```python
from build123d import *

# Parameters (mm, degrees)
BOSS_EXTRUDE1_DEPTH      = 30
BOSS_EXTRUDE1_DEPTH_BACK = 70
CUT_EXTRUDE1_REACH       = 92
SKETCH2_R                = 4.5
SKETCH2_R_2              = 5.1
SKETCH2_R_3              = 3.8
SKETCH5_W                = 20
SKETCH5_H                = 20
CUT_EXTRUDE2_DEPTH       = 91
CUT_EXTRUDE3_REACH       = 92
SKETCH7_W                = 20
SKETCH7_H                = 20
SKETCH8_R                = 5
SKETCH8_R_2              = 4.1
SKETCH8_R_3              = 3.8
CUT_EXTRUDE6_DEPTH       = 10
SKETCH9_W                = 20
SKETCH9_H                = 20
SKETCH9_W_2              = 3
SKETCH9_H_2              = 3
CUT_EXTRUDE7_DEPTH       = 81
BOSS_EXTRUDE2_DEPTH      = 80


with BuildPart() as part:
    # Sketch1 → Boss-Extrude1 (new body, two sides)
    with BuildSketch(Plane(origin=(0, 0, 0), x_dir=(1, 0, 0), z_dir=(0, 1, 0))) as boss_extrude1_sk:
        with BuildLine():
            Line((-25, 45), (25, 45))
            ThreePointArc((25, 45), (39.142135624, 39.142135624), (45, 25))
            Line((45, 25), (45, -25))
            ThreePointArc((45, -25), (39.142135624, -39.142135624), (25, -45))
            Line((25, -45), (-25, -45))
            ThreePointArc((-25, -45), (-39.142135624, -39.142135624), (-45, -25))
            Line((-45, -25), (-45, 25))
            ThreePointArc((-45, 25), (-39.142135624, 39.142135624), (-25, 45))
        make_face()
        with BuildLine():
            Line((-25, 35), (25, 35))
            ThreePointArc((25, 35), (32.071067812, 32.071067812), (35, 25))
            Line((35, 25), (35, -25))
            ThreePointArc((35, -25), (32.071067812, -32.071067812), (25, -35))
            Line((25, -35), (-25, -35))
            ThreePointArc((-25, -35), (-32.071067812, -32.071067812), (-35, -25))
            Line((-35, -25), (-35, 25))
            ThreePointArc((-35, 25), (-32.071067812, 32.071067812), (-25, 35))
        make_face(mode=Mode.SUBTRACT)
    extrude(amount=BOSS_EXTRUDE1_DEPTH)
    extrude(boss_extrude1_sk.sketch, amount=-BOSS_EXTRUDE1_DEPTH_BACK)

    # Sketch2 → Cut-Extrude1 (cut, up to next)
    with BuildSketch(Plane(origin=(45, 0, 0), x_dir=(0, 0, -1), z_dir=(1, 0, 0)), mode=Mode.PRIVATE) as cut_extrude1_sk1:
        with Locations((-0.001556395, 0)):
            Circle(SKETCH2_R)
    cut_extrude1_tool1 = extrude(cut_extrude1_sk1.sketch, amount=-CUT_EXTRUDE1_REACH, mode=Mode.PRIVATE) & part.part
    add(cut_extrude1_tool1.solids().sort_by_distance((45, 0, 0.001556))[0], mode=Mode.SUBTRACT)
    # Sketch2 → Cut-Extrude1 (cut, up to next)
    with BuildSketch(Plane(origin=(45, 0, 0), x_dir=(0, 0, -1), z_dir=(1, 0, 0)), mode=Mode.PRIVATE) as cut_extrude1_sk2:
        with Locations((-0.001556395, -35)):
            Circle(SKETCH2_R_2)
    cut_extrude1_tool2 = extrude(cut_extrude1_sk2.sketch, amount=-CUT_EXTRUDE1_REACH, mode=Mode.PRIVATE) & part.part
    add(cut_extrude1_tool2.solids().sort_by_distance((45, -35, 0.001556))[0], mode=Mode.SUBTRACT)
    # Sketch2 → Cut-Extrude1 (cut, up to next)
    with BuildSketch(Plane(origin=(45, 0, 0), x_dir=(0, 0, -1), z_dir=(1, 0, 0)), mode=Mode.PRIVATE) as cut_extrude1_sk3:
        with Locations((15.998443605, -35)):
            Circle(SKETCH2_R_3)
    cut_extrude1_tool3 = extrude(cut_extrude1_sk3.sketch, amount=-CUT_EXTRUDE1_REACH, mode=Mode.PRIVATE) & part.part
    add(cut_extrude1_tool3.solids().sort_by_distance((45, -35, -15.998444))[0], mode=Mode.SUBTRACT)
    # Sketch2 → Cut-Extrude1 (cut, up to next)
    with BuildSketch(Plane(origin=(45, 0, 0), x_dir=(0, 0, -1), z_dir=(1, 0, 0)), mode=Mode.PRIVATE) as cut_extrude1_sk4:
        with Locations((-16.001556395, -35)):
            Circle(SKETCH2_R_3)
    cut_extrude1_tool4 = extrude(cut_extrude1_sk4.sketch, amount=-CUT_EXTRUDE1_REACH, mode=Mode.PRIVATE) & part.part
    add(cut_extrude1_tool4.solids().sort_by_distance((45, -35, 16.001556))[0], mode=Mode.SUBTRACT)
    # Sketch2 → Cut-Extrude1 (cut, up to next)
    with BuildSketch(Plane(origin=(45, 0, 0), x_dir=(0, 0, -1), z_dir=(1, 0, 0)), mode=Mode.PRIVATE) as cut_extrude1_sk5:
        with BuildLine():
            ThreePointArc((20.848443603, 0), (18.248443605, 2.599999998), (15.648443602, 0))
            ThreePointArc((15.648443602, 0), (18.248443605, -2.600000003), (20.848443603, 0))
        make_face()
    cut_extrude1_tool5 = extrude(cut_extrude1_sk5.sketch, amount=-CUT_EXTRUDE1_REACH, mode=Mode.PRIVATE) & part.part
    add(cut_extrude1_tool5.solids().sort_by_distance((45, 0, -18.248444))[0], mode=Mode.SUBTRACT)
    # Sketch2 → Cut-Extrude1 (cut, up to next)
    with BuildSketch(Plane(origin=(45, 0, 0), x_dir=(0, 0, -1), z_dir=(1, 0, 0)), mode=Mode.PRIVATE) as cut_extrude1_sk6:
        with BuildLine():
            ThreePointArc((-15.651556392, 0), (-18.251556395, 2.600000003), (-20.851556393, 0))
            ThreePointArc((-20.851556393, 0), (-18.251556395, -2.599999997), (-15.651556392, 0))
        make_face()
    cut_extrude1_tool6 = extrude(cut_extrude1_sk6.sketch, amount=-CUT_EXTRUDE1_REACH, mode=Mode.PRIVATE) & part.part
    add(cut_extrude1_tool6.solids().sort_by_distance((45, 0, 18.251556))[0], mode=Mode.SUBTRACT)

    # Sketch5 → Cut-Extrude2 (cut, through all)
    with BuildSketch(Plane(origin=(45, 0, 0), x_dir=(0, 0, -1), z_dir=(1, 0, 0))):
        with Locations((35, 20)):
            Rectangle(SKETCH5_W, SKETCH5_H)
    extrude(amount=-CUT_EXTRUDE2_DEPTH, mode=Mode.SUBTRACT)

    # Sketch7 → Cut-Extrude3 (cut, up to next)
    with BuildSketch(Plane.XY.offset(45), mode=Mode.PRIVATE) as cut_extrude3_sk1:
        with Locations((-35, 20)):
            Rectangle(SKETCH7_W, SKETCH7_H)
    cut_extrude3_tool1 = extrude(cut_extrude3_sk1.sketch, amount=-CUT_EXTRUDE3_REACH, mode=Mode.PRIVATE) & part.part
    add(cut_extrude3_tool1.solids().sort_by_distance((-35, 20, 45))[0], mode=Mode.SUBTRACT)

    # Sketch8 → Cut-Extrude6 (cut)
    with BuildSketch(Plane.XY.offset(45)):
        with Locations((640, -50.6)):
            Circle(SKETCH8_R)
        with Locations((640, -15.6)):
            Circle(SKETCH8_R)
        with Locations((0, -15.6)):
            Circle(SKETCH8_R_2)
        with Locations((0, -50.6)):
            Circle(SKETCH8_R)
        with Locations((-16, -50.6)):
            Circle(SKETCH8_R_3)
        with Locations((16, -50.6)):
            Circle(SKETCH8_R_3)
        with BuildLine():
            ThreePointArc((-15.649999997, -15.6), (-18.25, -12.999999997), (-20.849999998, -15.6))
            ThreePointArc((-20.849999998, -15.6), (-18.25, -18.199999997), (-15.649999997, -15.6))
        make_face()
        with BuildLine():
            ThreePointArc((20.849999998, -15.6), (18.25, -13.000000002), (15.649999997, -15.6))
            ThreePointArc((15.649999997, -15.6), (18.25, -18.200000003), (20.849999998, -15.6))
        make_face()
    extrude(amount=-CUT_EXTRUDE6_DEPTH, mode=Mode.SUBTRACT)

    # Sketch9 → Cut-Extrude7 (cut, through all)
    with BuildSketch(Plane(origin=(0, 10, 0), x_dir=(1, 0, 0), z_dir=(0, 1, 0))):
        with Locations((-35, 35)):
            Rectangle(SKETCH9_W, SKETCH9_H)
        with Locations((-36.5, 15)):
            Rectangle(SKETCH9_W_2, SKETCH9_H)
        with Locations((-15, 36.5)):
            Rectangle(SKETCH9_W, SKETCH9_H_2)
    extrude(amount=-CUT_EXTRUDE7_DEPTH, mode=Mode.SUBTRACT)

    # Sketch10 → Boss-Extrude2 (add)
    with BuildSketch(Plane(origin=(0, 10, 0), x_dir=(1, 0, 0), z_dir=(0, 1, 0))):
        with BuildLine():
            Line((-25, 45), (-25, 25))
            Line((-25, 25), (-45, 25))
            Line((-45, 25), (-45, 15))
            Line((-45, 15), (-25, 15))
            ThreePointArc((-25, 15), (-17.928932188, 17.928932188), (-15, 25))
            Line((-15, 25), (-15, 45))
            Line((-15, 45), (-25, 45))
        make_face()
    extrude(amount=-BOSS_EXTRUDE2_DEPTH)


solid = part.part
```
Verification items for the finished model (mm, model axes). A direction names the side the tool comes from. Coordinates: 2 decimals unless noted, no trailing zeros. Write each loop counter-clockwise with the first axis right and the second up, starting at its lowest first coordinate (ties: lowest second). Pieces come first, ordered by that corner, then holes. Notation, with made-up numbers: M 44,-7 L 90,-7 A33 ccw 90,27 Z; hole C -34.5,-10 d2. An arc over 180 degrees is marked long. Answer as a JSON object with one key per item and string values. Group by question number.
(1) Tool access check on faces 1 (the face through (40.07, -31.232, 16.496)), 2 (the face through (39.297, -19.3, 38.986)), 3 (the face through (-20, 10, -20)), 4 (the face through (-15, -29, -31)), 5 (the face through (-1.08, -55.48, 40.07)). Record the directions out of +Z, -Z, +X, -X, +Y, -Y that give a thin tool (end or side, any length) a straight path to the whole face; none if there is none.
(2) Cross-section at A-A, the plane x = 9. Record the cut outline in (y, z).
(3) Cross-section at C-C, the plane x = 0. Record the cut outline in (y, z).
(4) Material ranges on line 1 (Y direction, x = 0, z = 42.25); line 2 (Z direction, x = 13.5, y = -4.5), recorded low to high.
(5) Release check for a two-part mould opening along X. For faces 6 (the face through (45, -19, 0)), 7 (the face through (15.51, -46.83, 40.07)), 8 (the face through (36, 30, 23)) record: +X half, -X half, draft (parallel to the pull), parting line (faces both ways), or undercut.
(6) Cross-section at D-D, the plane z = -17. Record the cut outline in (x, y).
(7) Gauge pin test, flat ends, axial feed: pin 1 (12 mm diameter, centred on y = -13, z = -34.5, fed in from +X); pin 2 (6 mm diameter, centred on x = -35.5, y = -47, fed in from -Z); pin 3 (10 mm diameter, centred on y = -29.5, z = -36.5, fed in from -X). Record the tip position at first contact, or that the pin passes through.
(8) Cross-section at B-B, the plane y = -61. Record the cut outline in (x, z), and give its area (3 significant figures).
Reply:
{
 "1": {"face 1": "+X", "face 2": "+Z, +X, +Y, -Y", "face 3": "-Z, -X, +Y", "face 4": "+Y, -Y", "face 5": "+Z"},
 "2": {"outline": "M -70,-45 L 10,-45 L 10,-35 L -70,-35 Z; M -70,35 L 30,35 L 30,45 L -70,45 Z"},
 "3": {"outline": "M -70,-45 L 10,-45 L 10,-35 L -70,-35 Z; M -70,35 L -55.6,35 L -55.6,45 L -70,45 Z; M -45.6,35 L -19.7,35 L -19.7,45 L -45.6,45 Z; M -11.5,35 L 30,35 L 30,45 L -11.5,45 Z"},
 "4": {"line 1": "-70 to -55.6, -45.6 to -19.7, -11.5 to 30", "line 2": "-45 to -35, 35 to 45"},
 "5": {"face 6": "+X half", "face 7": "undercut", "face 8": "draft"},
 "6": {"outline": "M -45,-70 L -19,-70 L -19,10 L -45,10 Z; M 35,-70 L 45,-70 L 45,-38.67 L 35,-38.67 Z; M 35,-31.33 L 45,-31.33 L 45,-2.28 L 35,-2.28 Z; M 35,2.28 L 45,2.28 L 45,30 L 35,30 Z"},
 "7": {"pin 1": "x = 44.69", "pin 2": "z = -25", "pin 3": "x = -25"},
 "8": {"outline": "M -45,-25 L -25,-25 L -25,-45 L 25,-45 A20 ccw 45,-25 L 45,25 A20 ccw 25,45 L -25,45 A20 ccw -45,25 Z; hole M -38,-15 L -25,-15 A10 cw -15,-25 L -15,-38 L -5,-38 L -5,-35 L 25,-35 A10 ccw 35,-25 L 35,25 A10 ccw 25,35 L -25,35 A10 ccw -35,25 L -35,-5 L -38,-5 Z", "area": "2,930 mm²"}
}
